Input: part model. Units: mm. Frame: model coordinates. Coordinates: 2 decimals unless noted, no trailing zeros. Loops run counter-clockwise (first coordinate to the right, second up) from the corner with the lowest first, then second, coordinate; pieces in that order, holes last.
```python
from build123d import *


with BuildPart() as part:
    # Esquisse1 → Révolution1 (revolve)
    with BuildSketch(Plane.XY):
        with BuildLine():
            Line((-100, 0), (0, 0))
            Line((0, 0), (0, 3.5))
            ThreePointArc((0, 3.5), (-0.439339828, 4.560660172), (-1.5, 5))
            Line((-1.5, 5), (-70, 5))
            Line((-70, 5), (-70, 4.999))
            Line((-70, 4.999), (-99, 4.999))
            Line((-99, 4.999), (-100, 3.999))
            Line((-100, 3.999), (-100, 0))
        make_face()
    revolve(axis=Axis((-100, 0, 0), (1, 0, 0)))


solid = part.part
```
Item 1: Line query: L1, parallel to Z at x = -6, y = -3; L2, parallel to Z at x = -77.5, y = 4; L3, parallel to Y at x = -17, z = -2.25. Output: solid intervals per line, ascending.
Result:
L1: z = -4 to 4
L2: z = -3 to 3
L3: y = -4.47 to 4.47
Item 2: Contact query for flat-ended pins moving along their axis: P1, Ø1, axis at y = 4, z = -2, coming from the +X side; P2, Ø3, axis at x = -88.5, y = -3, coming from the -Z side; P3, Ø2, axis at x = -58.5, z = -2.5, coming from the +Y side. Output: stop coordinate, or through.
Result:
P1: stops at x = -0.08
P2: stops at z = -4.77
P3: stops at y = 4.77
Item 3: Section query A-A (x = -12). Output: boundary loops of the cut face in (y, z).
Result:
outline: circle Ø10 at (0, 0)
